Geometry check sheet. Reference: the model listing, model coordinates, mm. A direction names the side the tool comes from. Coordinates: 2 decimals unless noted, no trailing zeros. Write each loop counter-clockwise with the first axis right and the second up, starting at its lowest first coordinate (ties: lowest second). Pieces come first, ordered by that corner, then holes.
from build123d import *

# Parameters (mm, degrees)
F0_R     = 1.5
F1_DEPTH = 5
F2_W     = 1
F2_H     = 6
F3_DEPTH = 1
F5_DEPTH = 15
F6_SIZE  = 0.4


with BuildPart() as f1:
    # F0 (on Front) → F1 (new body)
    with BuildSketch(Plane.XZ):
        Circle(F0_R)
    extrude(amount=F1_DEPTH)

    # F2 (on face) → F3 (join)
    with BuildSketch(Plane.XZ.offset(5)):
        Rectangle(F2_W, F2_H)
    extrude(amount=F3_DEPTH)

    # F4 (on face) → F5 (join)
    with BuildSketch(Plane.XZ.offset(6)):
        Polygon((0, 2.735806), (-0.5, 0), (0, -2.735806), (0.5, 0), align=None)
    extrude(amount=F5_DEPTH)

    # F6
    f6_edges = [f1.edges().sort_by_distance(p)[0] for p in [
        (0.25, -21, 1.367903),
        (0.25, -21, -1.367903),
        (-0.25, -21, 1.367903),
        (-0.25, -21, -1.367903),
    ]]
    chamfer(f6_edges, length=F6_SIZE)


solid = f1.part
1. Thickness scan on line 1 along Y through (x, z) = (0.2, 1.9); line 2 along X through (y, z) = (-5.5, -1.95); line 3 along X through (y, z) = (-7.25, 0.6). Record the ranges inside material, lowest first.
Computed values:
line 1: y = -6 to -5
line 2: x = -0.5 to 0.5
line 3: x = -0.39 to 0.39
2. Sectioned sample at B-B, the plane z = 2.3. Record the boundary of the cut face in (x, y), and give its area (3 significant figures).
Computed values:
outline: (-0.5, -6) - (-0.08, -6) - (-0.08, -20.6) - (0, -20.68) - (0.08, -20.6) - (0.08, -6) - (0.5, -6) - (0.5, -5) - (-0.5, -5) - close
area: 3.33 mm2
3. Sectioned sample at A-A, the plane y = -16. Record the boundary of the cut face in (x, z).
Computed values:
outline: (-0.5, 0) - (0, -2.74) - (0.5, 0) - (0, 2.74) - close
4. Access from +Z, -Z, +X, -X, +Y, -Y to the whole of each face (thin tool, end or side, straight path). Record for faces 1 (the flat face through (-0.5, -5.5, 0)), 2 (the flat face through (-0.247, -13.198, 1.387)), 3 (the flat face through (1, -5, 0)), 4 (the flat face through (-0.3, -6, -2.1)).
Computed values:
face 1: +Z, -Z, -X, -Y
face 2: +Z, -X, -Y
face 3: +Z, -Z, +X, -Y
face 4: -Z, -Y
5. Gauge pin test, flat ends, axial feed: pin 1 Ø0.5 at (x, z) = (-1, -0.5) entering from -Y; pin 2 Ø1.1 at (x, z) = (0, 2) entering from -Y; pin 3 Ø1.5 at (y, z) = (-13, 1.5) entering from -X. Record the tip position at first contact, or that the pin passes through.
Computed values:
pin 1: stops at y = -5
pin 2: stops at y = -20.83
pin 3: stops at x = -0.36
6. Sectioned sample at C-C, the plane x = 0.8. Record the boundary of the cut face in (y, z).
Computed values:
outline: (-5, -1.27) - (0, -1.27) - (0, 1.27) - (-5, 1.27) - close
7. Sectioned sample at D-D, the plane z = 1.1. Record the boundary of the cut face in (x, y), and give its area (3 significant figures).
Computed values:
outline: (-1.02, -5) - (-0.5, -5) - (-0.5, -6) - (-0.3, -6) - (-0.3, -20.6) - (0, -20.89) - (0.3, -20.6) - (0.3, -6) - (0.5, -6) - (0.5, -5) - (1.02, -5) - (1.02, 0) - (-1.02, 0) - close
area: 20.0 mm2
